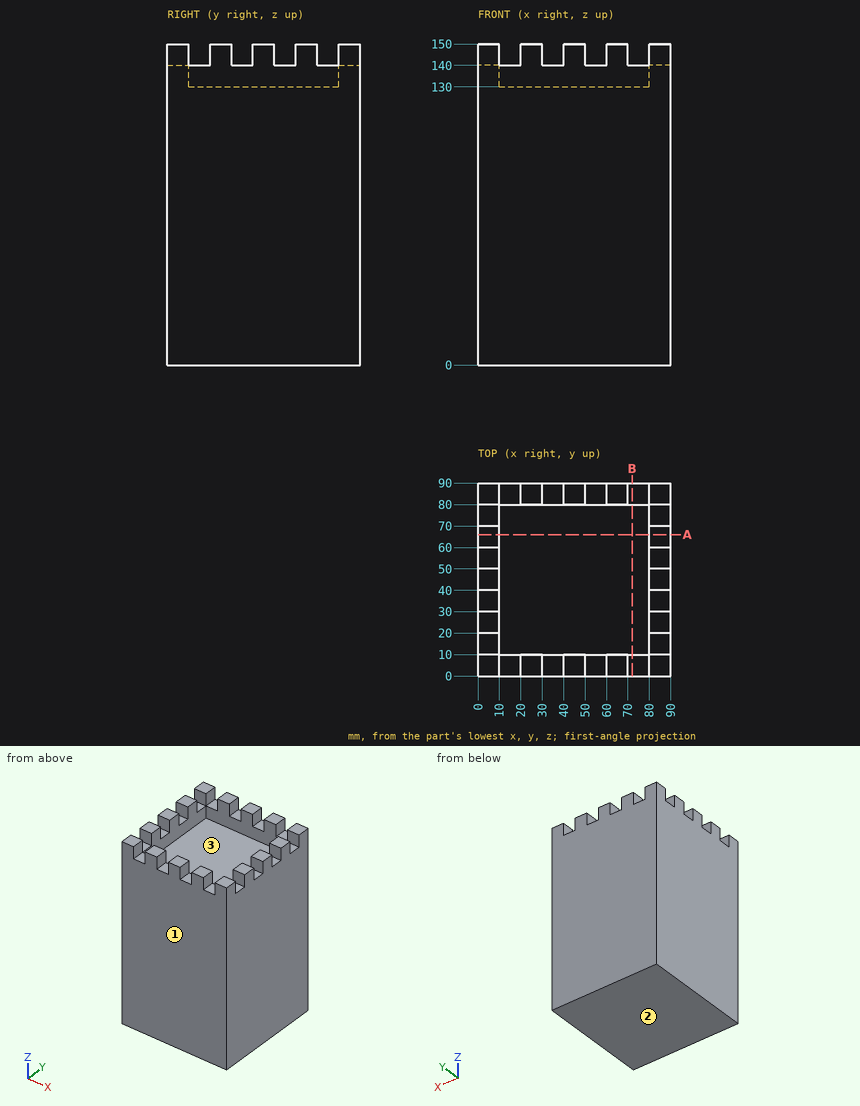
Design review of the part shown in the three views and the two pictorial views. Dimensions are in mm from the part's minimum x, y and z. Round coordinates to 2 decimals unless told otherwise and drop trailing zeros. Loops run counter-clockwise (first coordinate to the right, second up) from the corner with the lowest first, then second, coordinate; pieces in that order, holes last.
Q1. Mouldability with a two-part tool opening along Y and no side actions: class the marked faces 1, 2 and 3 as +Y half, -Y half, draft (parallel to the pull), parting line (faces both ways), or undercut.
Result sheet:
face 1: -Y half
face 2: draft
face 3: undercut
Q2. Insertion check: pin 1 Ø8 at (x, y) = (84, 35.5) entering from +Z; pin 2 Ø21 at (x, y) = (42, 36.5) entering from +Z. Each pin has a flat end and moves straight along its axis. Give the tip position at first contact, or say it passes through.
Result sheet:
pin 1: stops at z = 140
pin 2: stops at z = 130
Q3. To check wall thickness, follow line 1 along Y through (x, z) = (59.5, 135.5); line 2 along Z through (x, y) = (14.5, 58); line 3 along Z through (x, y) = (56.5, 5). State the ranges of each line that lie inside material, in increasing order.
Result sheet:
line 1: y = 0 to 10, 80 to 90
line 2: z = 0 to 130
line 3: z = 0 to 140
Q4. Add section B-B on x = 72. Write out the cut boundary in (y, z), plus the area to 3 significant figures.
Result sheet:
outline: (0, 0) - (90, 0) - (90, 140) - (80, 140) - (80, 130) - (10, 130) - (10, 140) - (0, 140) - close
area: 11,900 mm2
Q5. Add section A-A on y = 66. Write out the cut boundary in (x, z).
Result sheet:
outline: (0, 0) - (90, 0) - (90, 150) - (80, 150) - (80, 130) - (10, 130) - (10, 150) - (0, 150) - close
